Could you check a few things on this drawing? It's one solid part, dimensions in mm from its lowest x, y, z. Round coordinates to 2 decimals unless told otherwise and drop trailing zeros. Write each loop counter-clockwise with the first axis right and the second up, starting at its lowest first coordinate (ties: lowest second). Pieces come first, ordered by that corner, then holes. Notation, with made-up numbers: (-32, 9) -> (-10, 9) arc R6 cw to (-10, 16) -> close; hole circle Ø9 at (42, -26). An arc over 180 degrees is marked (long way). Return JSON: item names as keys, results as strings.
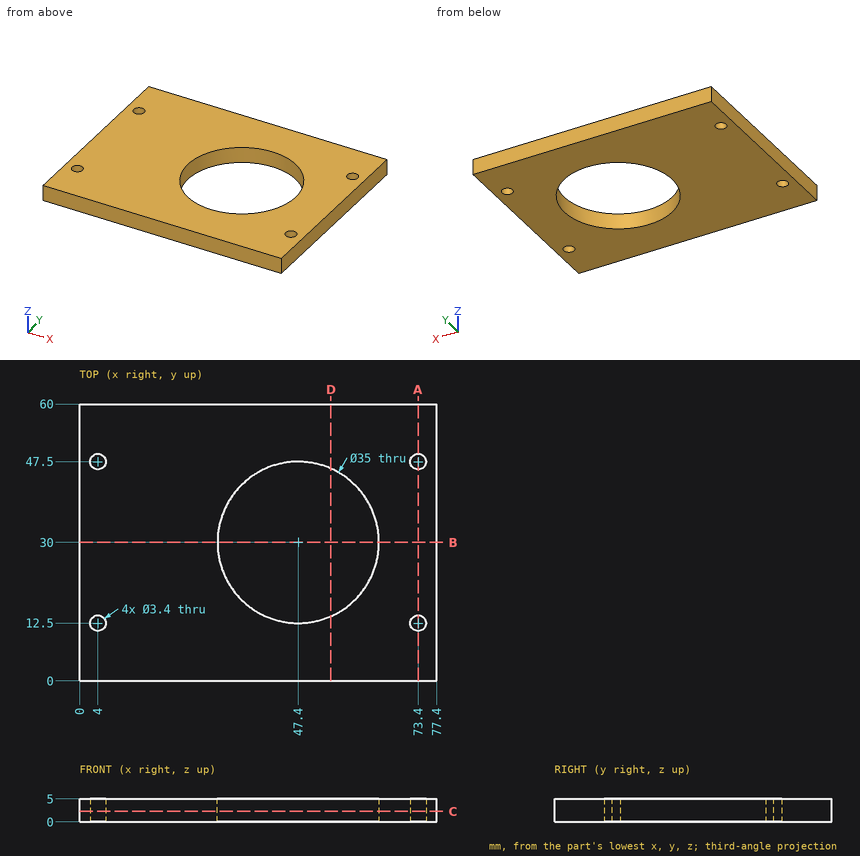
1) Will this pin go through, and if not, where does the flat tip stop? pin 1 Ø3 at (y, z) = (42.5, 2) entering from -X.
Return value:
{"pin 1": "x = 0"}
2) I want a section at A-A, the plane x = 73.4. Please give me the cut outline in (y, z), and give its area (3 significant figures).
Return value:
{"outline": "(0, 0) -> (10.8, 0) -> (10.8, 5) -> (0, 5) -> close; (14.2, 0) -> (45.8, 0) -> (45.8, 5) -> (14.2, 5) -> close; (49.2, 0) -> (60, 0) -> (60, 5) -> (49.2, 5) -> close", "area": "266 mm²"}
3) If I drill on probe 1 along Y at (x, z) = (4, 2.7); probe 2 along Y at (x, z) = (47.4, 2.35); probe 3 along X at (y, z) = (49, 0.5), over which ranges is the centre line in solid material (lowest first)? Write a range as [from, to].
Return value:
{"probe 1": "[0, 10.8], [14.2, 45.8], [49.2, 60]", "probe 2": "[0, 12.5], [47.5, 60]", "probe 3": "[0, 3.2], [4.8, 72.6], [74.2, 77.4]"}
4) I want a section at B-B, the plane y = 30. Please give me the cut outline in (x, z).
Return value:
{"outline": "(0, 0) -> (29.9, 0) -> (29.9, 5) -> (0, 5) -> close; (64.9, 0) -> (77.4, 0) -> (77.4, 5) -> (64.9, 5) -> close"}
5) I want a section at D-D, the plane x = 54.5. Please give me the cut outline in (y, z) (3 decimals).
Return value:
{"outline": "(0, 0) -> (14.005, 0) -> (14.005, 5) -> (0, 5) -> close; (45.995, 0) -> (60, 0) -> (60, 5) -> (45.995, 5) -> close"}
6) I want a section at C-C, the plane z = 2.3. Please give me the cut outline in (x, y), and give its area (3 significant figures).
Return value:
{"outline": "(0, 0) -> (77.4, 0) -> (77.4, 60) -> (0, 60) -> close; hole circle Ø3.4 at (4, 12.5); hole circle Ø3.4 at (4, 47.5); hole circle Ø35 at (47.4, 30); hole circle Ø3.4 at (73.4, 12.5); hole circle Ø3.4 at (73.4, 47.5)", "area": "3,650 mm²"}
